Build history of the part. All positions in model axes, mm. Round coordinates to 2 decimals unless told otherwise and drop trailing zeros. Write each loop counter-clockwise with the first axis right and the second up, starting at its lowest first coordinate (ties: lowest second). Pieces come first, ordered by that corner, then holes. Notation, with made-up numbers: (15, 54) -> (65, 54) arc R19 ccw to (65, 78) -> close; hole circle Ø6 at (-11, 83.5). An arc over 180 degrees is marked (long way). Answer in a Markdown table with one row per item.
```python
from build123d import *

# Parameters (mm, degrees)
F2_R     = 152.4
F2_R_2   = 151.9174
F5_R     = 152.4
F5_R_2   = 151.9174
F7_DEPTH = 711.2010001
F8_DEPTH = 457.2


with BuildPart() as f3:
    # F3: sweep along a path in F0
    with BuildLine(Plane.XZ) as f3_path:
        Line((0, 0), (0, 711.2))
    # F2 (on line) → F3 (sweep)
    with BuildSketch(Plane.XY):
        Circle(F2_R)
        Circle(F2_R_2, mode=Mode.SUBTRACT)
    sweep(path=f3_path.line)

    # F6: sweep along a path in F0
    with BuildLine(Plane.XZ) as f6_path:
        Line((0, 254), (323.2892203585, 577.2892203585))
    # F5 (on line) → F6 (sweep)
    with BuildSketch(Plane(origin=(450.2892203585, 0, 450.2892203585), x_dir=(0, 1, 0), z_dir=(0.7071067812, 0, 0.7071067812))):
        with Locations((0, 179.6051224214)):
            Circle(F5_R)
        with Locations((0, 179.6051224214)):
            Circle(F5_R_2, mode=Mode.SUBTRACT)
    sweep(path=f6_path.line)

    # F2 (on line) → F7 (cut, through all)
    with BuildSketch(Plane.XY):
        Circle(F2_R_2)
    extrude(amount=F7_DEPTH, mode=Mode.SUBTRACT)

    # F5 (on line) → F8 (cut)
    with BuildSketch(Plane(origin=(450.2892203585, 0, 450.2892203585), x_dir=(0, 1, 0), z_dir=(0.7071067812, 0, 0.7071067812))):
        with Locations((0, 179.6051224214)):
            Circle(F5_R_2)
    extrude(amount=-F8_DEPTH, mode=Mode.SUBTRACT)


solid = f3.part
```
Q1. Saw through at A-A on y = 14. Write the cut outline in (x, z).
A:
| item | result |
|---|---|
| outline | (-151.76, 0) -> (-151.27, 0) -> (-151.27, 711.2) -> (-151.76, 711.2) -> close; (151.27, 0) -> (151.76, 0) -> (151.76, 191.14) -> (430.6, 469.98) -> (430.25, 470.32) -> (151.27, 191.34) -> close; (151.27, 619.2) -> (216.32, 684.25) -> (215.98, 684.6) -> (151.76, 620.37) -> (151.76, 711.2) -> (151.27, 711.2) -> close |
Q2. Saw through at D-D on y = 57. Write the cut outline in (x, z).
A:
| item | result |
|---|---|
| outline | (-141.34, 0) -> (-140.82, 0) -> (-140.82, 711.2) -> (-141.34, 711.2) -> close; (140.82, 0) -> (141.34, 0) -> (141.34, 195.46) -> (423.23, 477.35) -> (422.86, 477.72) -> (140.82, 195.67) -> close; (140.82, 593.97) -> (223.72, 676.86) -> (223.35, 677.23) -> (141.34, 595.22) -> (141.34, 711.2) -> (140.82, 711.2) -> close |
Q3. Saw through at B-B on x = -71. Write the cut outline in (y, z).
A:
| item | result |
|---|---|
| outline | (-134.85, 0) -> (-134.31, 0) -> (-134.31, 711.2) -> (-134.85, 711.2) -> close; (134.31, 0) -> (134.85, 0) -> (134.85, 711.2) -> (134.31, 711.2) -> close |
Q4. Saw through at C-C on z = 148. Write the cut outline in (x, y), plus the area to 3 significant figures.
A:
| item | result |
|---|---|
| outline | circle Ø304.8 at (0, 0); hole circle Ø303.83 at (0, 0) |
| area | 461 mm² |
Q5. Drop flat-ended pins along their axis: P1, Ø5, axis at y = -45.5, z = 413, coming from the -X side; P2, Ø3, axis at x = 201, y = -55.5, coming from the -Z side; P3, Ø8, axis at y = -34, z = 224.5, coming from the -X side. Give the stop position or say it passes through.
A:
| item | result |
|---|---|
| P1 | x = -146.21 |
| P2 | z = 252.56 |
| P3 | x = -149.42 |
Q6. Wall check: line 1 (Y direction, x = 0, z = 329); line 2 (Y direction, x = 104, z = 241.5); line 3 (X direction, y = 75, z = 229.5). Give the ranges that are in metal, low to high. Write a range as [from, to].
A:
| item | result |
|---|---|
| line 1 | [-152.4, -151.92], [151.92, 152.4] |
| line 2 | [-128.22, -127.64], [127.64, 128.22] |
| line 3 | [-132.67, -132.11], [162.34, 163.12] |
Q7. Two-plate mould, pull along Y, no slides. Class faces 1 (the cylindrical face through (304.696, -32.933, 348.961)), 2 (the cylindrical face through (-152.253, 6.701, 360.578)): released by +Y, released by -Y, zero draft, split by the parting line, or undercut.
A:
| item | result |
|---|---|
| face 1 | undercut |
| face 2 | split by the parting line |
